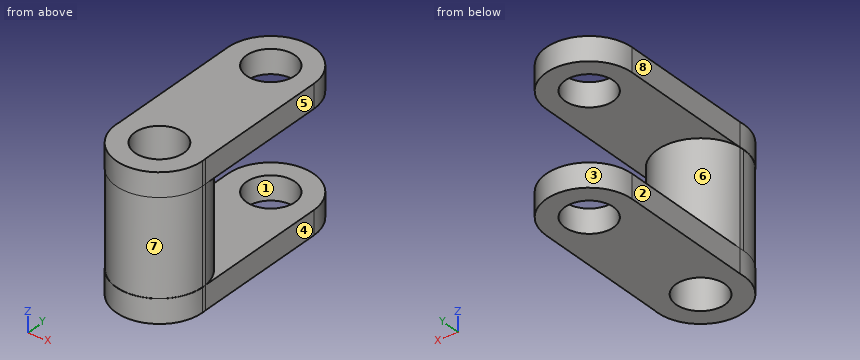
from build123d import *

# Parameters (mm, degrees)
F1_DEPTH = 76.2
F2_DEPTH = 25.4


with BuildPart() as f1:
    # F0 (on Top) → F1 (new body)
    with BuildSketch(Plane.XY):
        with BuildLine():
            Line((48.4909079969, -76.0845467448), (48.4909079969, -71.5253020613))
            ThreePointArc((48.4909079969, -71.5253020613), (2.4245455861, -29.7931171077), (-43.6418168247, -71.5253020613))
            Line((-43.6418168247, -71.5253020613), (-43.6418168247, -76.0845467448))
            Line((-43.6418168247, -76.0845467448), (-23.7078333656, -76.0845467448))
            ThreePointArc((-23.7078333656, -76.0845467448), (2.4245455861, -49.9521677931), (28.5569245378, -76.0845467448))
            Line((28.5569245378, -76.0845467448), (48.4909079969, -76.0845467448))
        make_face()
        with BuildLine():
            ThreePointArc((-43.6418168247, -76.0845467448), (2.4245455861, -122.1509091556), (48.4909079969, -76.0845467448))
            Line((48.4909079969, -76.0845467448), (28.5569245378, -76.0845467448))
            ThreePointArc((28.5569245378, -76.0845467448), (2.4245455861, -102.2169256965), (-23.7078333656, -76.0845467448))
            Line((-23.7078333656, -76.0845467448), (-43.6418168247, -76.0845467448))
        make_face()
    extrude(amount=F1_DEPTH)

    # F0 (on Top) → F2 (join)
    with BuildSketch(Plane.XY):
        with BuildLine():
            ThreePointArc((-23.5266864031, 76.5463635325), (2.4245455861, 102.4975955217), (28.3757775753, 76.5463635325))
            Line((28.3757775753, 76.5463635325), (48.4909079969, 76.5463635325))
            ThreePointArc((48.4909079969, 76.5463635325), (2.4245455861, 122.6127259433), (-43.6418168247, 76.5463635325))
            Line((-43.6418168247, 76.5463635325), (-23.5266864031, 76.5463635325))
        make_face()
        with BuildLine():
            Line((48.4909079969, 76.5463635325), (28.3757775753, 76.5463635325))
            ThreePointArc((28.3757775753, 76.5463635325), (2.4245455861, 50.5951315433), (-23.5266864031, 76.5463635325))
            Line((-23.5266864031, 76.5463635325), (-43.6418168247, 76.5463635325))
            Line((-43.6418168247, 76.5463635325), (-43.6418168247, -71.5253020613))
            ThreePointArc((-43.6418168247, -71.5253020613), (2.4245455861, -29.7931171077), (48.4909079969, -71.5253020613))
            Line((48.4909079969, -71.5253020613), (48.4909079969, 76.5463635325))
        make_face()
        with BuildLine():
            ThreePointArc((48.7159752232, -76.0845467448), (48.6596741791, -73.8021484809), (48.4909079969, -71.5253020613))
            Line((48.4909079969, -71.5253020613), (48.4909079969, -76.0845467448))
            ThreePointArc((48.4909079969, -76.0845467448), (2.4245455861, -122.1509091556), (-43.6418168247, -76.0845467448))
            Line((-43.6418168247, -76.0845467448), (-43.6418168247, -71.5253020613))
            ThreePointArc((-43.6418168247, -71.5253020613), (0.1421473222, -122.3196753378), (48.7159752232, -76.0845467448))
        make_face()
        with BuildLine():
            Line((48.4909079969, -76.0845467448), (48.4909079969, -71.5253020613))
            ThreePointArc((48.4909079969, -71.5253020613), (2.4245455861, -29.7931171077), (-43.6418168247, -71.5253020613))
            Line((-43.6418168247, -71.5253020613), (-43.6418168247, -76.0845467448))
            Line((-43.6418168247, -76.0845467448), (-23.7078333656, -76.0845467448))
            ThreePointArc((-23.7078333656, -76.0845467448), (2.4245455861, -49.9521677931), (28.5569245378, -76.0845467448))
            Line((28.5569245378, -76.0845467448), (48.4909079969, -76.0845467448))
        make_face()
    extrude(amount=F2_DEPTH)

    # F3: F1 across face


with BuildPart() as f1_1:
    add(f1.part)
    add(f1.part.mirror(Plane(origin=(2.4245455861, -75.8742165299, 76.2), x_dir=(1, 0, 0), z_dir=(0, 0, 1))))


solid = f1_1.part
Can you work these out from the model? Positions are in its coordinate system, mm. Face numbers are marked on the shaded views. A direction names the side the tool comes from. Coordinates: 2 decimals unless noted, no trailing zeros. Order: outer loops, then holes, each group sorted by start corner. A loop starts at its lowest first (then second) coordinate and runs counter-clockwise, first axis right, second up. Notation, with made-up numbers: (12, 13.5) - (60, 13.5) arc R23 ccw to (60, 41.5) - close; hole circle Ø6 at (67.25, 79.25). An arc over 180 degrees is marked (long way). Answer as a JSON object with one key per item and string values. Group by question number.
Q1. On a 3-axis mill with a long thin cutter (end or side, diameter ignored), from which of +Z, -Z, +X, -X, +Y, -Y can I reach the whole of each face in a straight line? I mean the marked faces 5, 6, 7 and 8. Say none if no direction works.
Q2. I need wall thicknesses on line 1 (Z direction, x = 40.5, y = 82); line 2 (X direction, y = 37, z = 136); line 3 (Y direction, x = -8, z = 105.5). Which ranges of each line are inside material? Lowest first, please. Write a range as from..to.
Q3. Imagine slicing it at C-C (x = 1.5). Please give me the cut outline in (y, z), and give its area (3 significant figures).
Q4. We'd pull the mould along X, two halves only. Please class the marked faces 1, 2, 3 and 4: +X half, -X half, draft (parallel to the pull), parting line (faces both ways), or undercut.
Q5. Imagine slicing it at B-B (y = 25). Please give me the cut outline in (x, z), and give its area (3 significant figures).
Q6. Will these pins go through, and if not, where does the flat tip stop? P1, Ø8, axis at y = -75, z = 102, coming from the +X side; P2, Ø20.5, axis at y = 1, z = 9, coming from the -X side; P3, Ø1, axis at x = 5.5, z = 19.5, coming from the -Y side.
Determined:
{
 "1": {"face 5": "+Z, -Z, +X, +Y", "face 6": "+Y", "face 7": "-Y", "face 8": "+Z, -Z, -X, +Y"},
 "2": {"line 1": "z = 0..25.4, 127..152.4", "line 2": "x = -43.64..48.49", "line 3": "y = -120.96..-100.05, -52.12..-30.98"},
 "3": {"outline": "(-122.37, 0) - (-102.2, 0) - (-102.2, 152.4) - (-122.37, 152.4) - (-122.37, 127) - (-122.14, 127) - (-122.14, 25.4) - (-122.37, 25.4) - close; (-49.97, 0) - (50.61, 0) - (50.61, 25.4) - (-29.8, 25.4) - (-29.8, 127) - (50.61, 127) - (50.61, 152.4) - (-49.97, 152.4) - close; (102.48, 0) - (122.6, 0) - (122.6, 25.4) - (102.48, 25.4) - close; (102.48, 127) - (122.6, 127) - (122.6, 152.4) - (102.48, 152.4) - close", "area": "11,200 mm2"},
 "4": {"face 1": "undercut", "face 2": "-X half", "face 3": "parting line", "face 4": "+X half"},
 "5": {"outline": "(-43.64, 0) - (48.49, 0) - (48.49, 25.4) - (-43.64, 25.4) - close; (-43.64, 127) - (48.49, 127) - (48.49, 152.4) - (-43.64, 152.4) - close", "area": "4,680 mm2"},
 "6": {"P1": "stops at x = 48.49", "P2": "stops at x = -43.64", "P3": "stops at y = -122.3"}
}
